Design review of the part shown in the three views and the two pictorial views. Dimensions are in mm from the part's minimum x, y and z. Round coordinates to 2 decimals unless told otherwise and drop trailing zeros. Loops run counter-clockwise (first coordinate to the right, second up) from the corner with the lowest first, then second, coordinate; pieces in that order, holes last.
1. Consider section C-C on x = 175.5. State the section outline as (y, z) points.
2. Consider section A-A on z = 135. State the section outline as (x, y) points.
3. Clearance check with flat-ended pins moving along their axes: pin 1 Ø5.5 at (x, z) = (7, 6.5) entering from -Y; pin 2 Ø2 at (x, z) = (184, 158.5) entering from +Y. State where each tip first meets the part, or that it passes through.
4. Consider section B-B on y = 6.25. State the section outline as (x, z) points, then the cut area to 3 significant figures.
5. To check wall thickness, follow line 1 along X through (y, z) = (4.1, 6.5); line 2 along Z through (x, y) = (7, 7.05); line 3 along Z through (x, y) = (7, 4.45). State the ranges of each line that lie inside material, in increasing order.
6. Draft analysis for pull direction X (two halves, no side actions). For the marked faces 1 and 2, state which applies: released by +X, released by -X, zero draft, split by the parting line, or undercut.
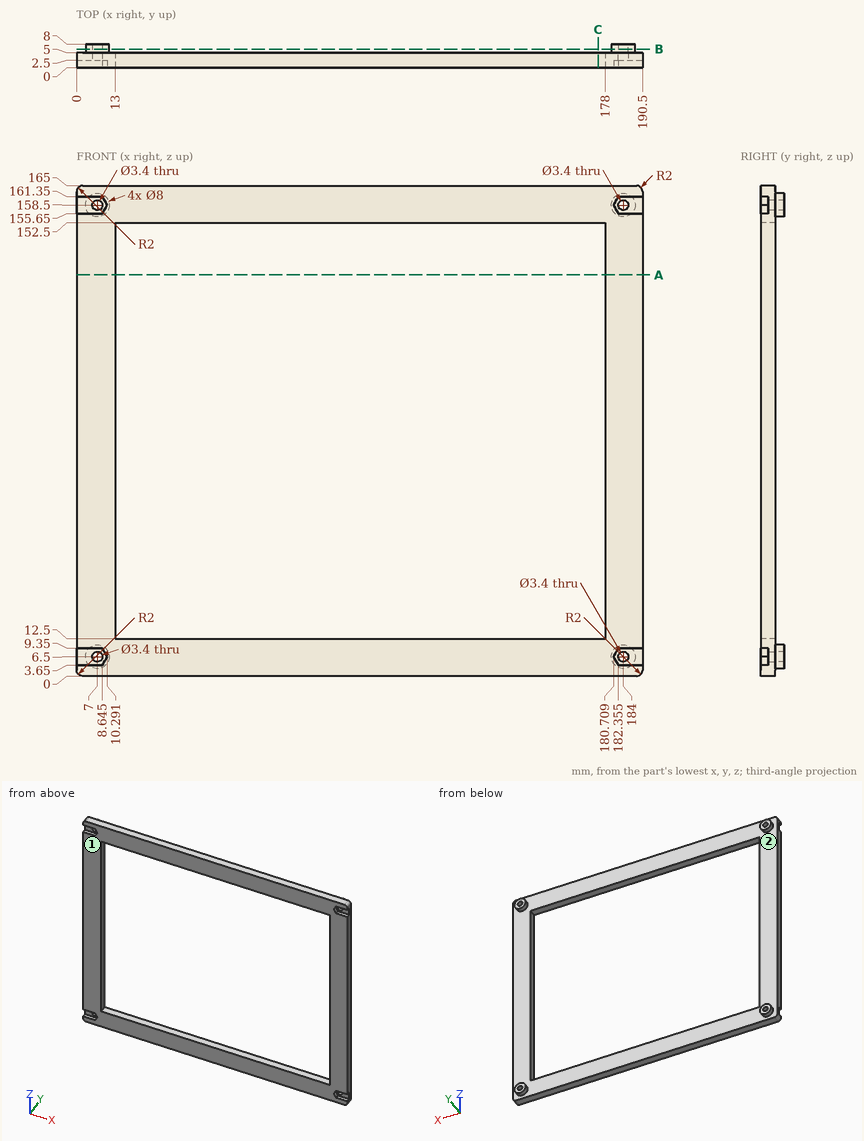
Resolved:
1. outline: (0, 0) - (5, 0) - (5, 12.5) - (0, 12.5) - close; (0, 152.5) - (5, 152.5) - (5, 165) - (0, 165) - close
2. outline: (0, 0) - (13, 0) - (13, 5) - (0, 5) - close; (178, 0) - (190.5, 0) - (190.5, 5) - (178, 5) - close
3. pin 1: stops at y = 2.5
3. pin 2: passes through
4. outline: circle Ø8 at (7, 6.5); circle Ø8 at (7, 158.5); circle Ø8 at (184, 6.5); circle Ø8 at (184, 158.5); hole circle Ø3.4 at (7, 6.5); hole circle Ø3.4 at (7, 158.5); hole circle Ø3.4 at (184, 6.5); hole circle Ø3.4 at (184, 158.5)
4. area: 165 mm2
5. line 1: x = 0 to 5.3, 8.7 to 182.3, 185.7 to 190.5
5. line 2: z = 2.5 to 4.8, 8.2 to 10.5, 154.5 to 156.8, 160.2 to 162.5
5. line 3: z = 0 to 4.8, 8.2 to 156.8, 160.2 to 165
6. face 1: zero draft
6. face 2: undercut
